Design review of the part built by this model. Coordinates are the model's own, in mm. Coordinates: 2 decimals unless noted, no trailing zeros. Loops run counter-clockwise (first coordinate to the right, second up) from the corner with the lowest first, then second, coordinate; pieces in that order, holes last. Notation, with made-up numbers: (38, 74) -> (89, 74) arc R35 cw to (89, 108) -> close; hole circle Ø3 at (-0.75, 52). An arc over 180 degrees is marked (long way). Use one line per item in the form item = value. Start each with the question number.
1. Consider section C-C (x = -25). State the section outline as (y, z) points.
2. Wall thickness on line 1 (Z direction, x = 30, y = 5.5); line 2 (Z direction, x = -70, y = 2.75); line 3 (Z direction, x = -25, y = 3.75): over which ranges is each line inside the solid? List them lowest first. Write a range as from..to.
3. Consider section B-B (z = 110). State the section outline as (x, y) points, then the cut area to 3 significant figures.
4. Consider section A-A (x = -70). State the section outline as (y, z) points, then the cut area to 3 significant figures.
Autodesk Inventor part; units mm, degrees
ref_plane "YZ Plane" through (0, 0, 0) normal (1, 0, 0) x (0, 1, 0)
ref_plane "XZ Plane" through (0, 0, 0) normal (0, 1, 0) x (-1, 0, 0)
ref_plane "XY Plane" through (0, 0, 0) normal (0, 0, 1) x (1, 0, 0)
sketch "Block1" plane through (0, 0, 0) normal (0, 0, 1) x (1, 0, 0)
  line L0 (-75.22, -185.22) -> (-75.22, 35.22)
  line L1 (-75.22, 35.22) -> (35.22, 35.22)
  line L2 (35.22, 35.22) -> (35.22, -185.22)
  line L3 (35.22, -185.22) -> (-75.22, -185.22)
  circle A0 centre (-70, -180) radius 2.72
  circle A1 centre (-25, -177.5) radius 2.72
  circle A2 centre (30, -180) radius 2.72
  circle A3 centre (-25, 30) radius 2.72
  circle A4 centre (-70, 30) radius 2.72
  circle A5 centre (30, -40) radius 2.72
  circle A6 centre (30, -110) radius 2.72
  circle A7 centre (-25, -110) radius 5.22
  circle A8 centre (-25, -40) radius 5.22
  circle A9 centre (30, 30) radius 2.72
  point P0 (-15, -74.8437)
sketch "Sketch1" plane through (0, 0, 0) normal (0, 1, 0) x (-1, 0, 0)
  line L0 (0, 0) -> (75, 0)
  line L1 (75, 0) -> (75, 185)
  line L2 (75, 185) -> (0, 185)
  circle A0 centre (25, 110) radius 5
  circle A1 centre (25, 40) radius 5
  line L3 (75, 185) -> (100, 185)
  line L4 (75, 0) -> (100, 0)
  line L5 (0, 0) -> (-35, 0)
  line L6 (-35, 0) -> (-35, 185)
  line L7 (-35, 185) -> (0, 185)
  line L8 (106.8257, 75) -> (-45.4509, 75)
  line L9 (-35, 0) -> (75, 0)
  line L10 (75, 0) -> (75, -35)
  line L11 (75, -35) -> (-35, -35)
  line L12 (-35, -35) -> (-35, 0)
  circle A2 centre (-30, 180) radius 2.5
  circle A3 centre (70, 180) radius 2.5
  circle A4 centre (-30, -30) radius 2.5
  circle A5 centre (70, -30) radius 2.5
  circle A6 centre (-30, 110) radius 2.5
  circle A7 centre (-30, 40) radius 2.5
  circle A8 centre (25, 177.5) radius 2.5
  circle A9 centre (25, -30) radius 2.5
  dimension "d5" = 10
  dimension "d9" = 70
  dimension "d13" = 35
  dimension "d14" = 50
  dimension "d17" = 75
  dimension "d18" = 185
  dimension "d19" = 35
  dimension "d22" = 5
  dimension "d23" = 5
  dimension "d24" = 5
  dimension "d25" = 5
  dimension "d26" = 5
  dimension "d27" = 5
  dimension "d28" = 5
  dimension "d29" = 5
  dimension "d30" = 5
  dimension "d31" = 5
  dimension "d32" = 5
  dimension "d33" = 75
  dimension "d34" = 5
  dimension "d35" = 75
  dimension "d36" = 5
  dimension "d37" = 5
  dimension "d38" = 5
  dimension "d39" = 5
  dimension "d42" = 5
  dimension "d43" = 50
  dimension "d46" = 5
  dimension "d47" = 5
  dimension "d48" = 50
extrude "Extrusion5" add sketch "Sketch1" along normal blind 10
sketch "Sketch2" plane through (0, 10, 0) normal (0, 1, 0) x (1, 0, 0)
  circle A0 centre (-25, -40) radius 5
  circle A1 centre (-25, -110) radius 5
  circle A2 centre (-25, -177.5) radius 2.5
  circle A3 centre (30, -40) radius 2.5
  circle A4 centre (30, -110) radius 2.5
  circle A5 centre (-70, -180) radius 2.5
  circle A6 centre (30, -180) radius 2.5
  circle A7 centre (-25, 30) radius 2.5
  circle A8 centre (-70, 30) radius 2.5
  circle A9 centre (30, 30) radius 2.5
  line L0 (35, -185) -> (35, 35)
  line L1 (35, 35) -> (-75, 35)
  line L2 (-75, 35) -> (-75, -185)
  line L3 (-75, -185) -> (35, -185)
  point P0 (0, 0)
sketch "DXF" plane through (0, 0, 0) normal (0, 1, 0) x (-1, 0, 0)
  point P0 (0, 0)
properties part number "shaft_cover"
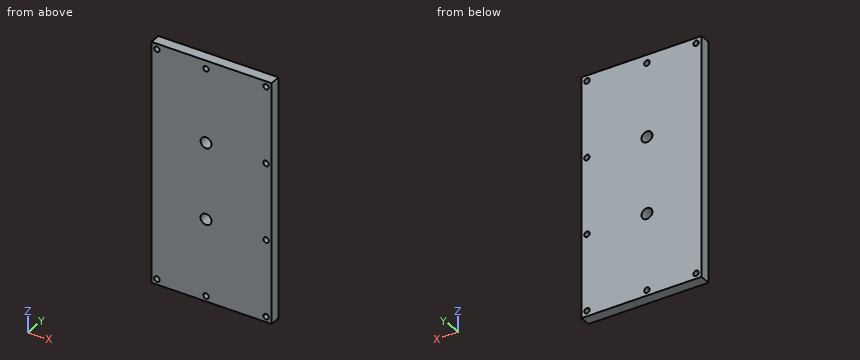
Geometry check:
q1.outline = (0, -35) -> (10, -35) -> (10, -32.5) -> (0, -32.5) -> close; (0, -27.5) -> (10, -27.5) -> (10, 35) -> (0, 35) -> close; (0, 45) -> (10, 45) -> (10, 105) -> (0, 105) -> close; (0, 115) -> (10, 115) -> (10, 175) -> (0, 175) -> close; (0, 180) -> (10, 180) -> (10, 185) -> (0, 185) -> close
q2.line_1 = -35..-32.5, -27.5..37.5, 42.5..107.5, 112.5..177.5, 182.5..185
q2.line_2 = -35..-32.5, -27.5..177.5, 182.5..185
q2.line_3 = -35..-32.5, -27.5..35, 45..105, 115..175, 180..185
q3.outline = (-75, 0) -> (-30, 0) -> (-30, 10) -> (-75, 10) -> close; (-20, 0) -> (27.5, 0) -> (27.5, 10) -> (-20, 10) -> close; (32.5, 0) -> (35, 0) -> (35, 10) -> (32.5, 10) -> close
q3.area = 950 mm²
q4.outline = (0, -35) -> (10, -35) -> (10, -32.5) -> (0, -32.5) -> close; (0, -27.5) -> (10, -27.5) -> (10, 177.5) -> (0, 177.5) -> close; (0, 182.5) -> (10, 182.5) -> (10, 185) -> (0, 185) -> close
q4.area = 2,100 mm²
